Can you work these out from the model? Positions are in its coordinate system, mm. A direction names the side the tool comes from. Round coordinates to 2 decimals unless told otherwise and drop trailing zeros. Loops run counter-clockwise (first coordinate to the right, second up) from the corner with the lowest first, then second, coordinate; pieces in that order, holes last.
from build123d import *

# Parameters (mm, degrees)
ESQUISSE1_W                                    = 408.5
ESQUISSE1_H                                    = 181
BOSS_EXTRU_1_DEPTH                             = 8
CHAMBRAGE_POUR_VIS_T_TE_RONDE_BOMB_2_COUNT     = 2
CHAMBRAGE_POUR_VIS_T_TE_RONDE_BOMB_2_PITCH     = 56
CHAMBRAGE_POUR_VIS_T_TE_RONDE_BOMB_3_COUNT     = 2
CHAMBRAGE_POUR_VIS_T_TE_RONDE_BOMB_3_PITCH     = 140
R_P_TITION_LIN_AIRE1_COUNT                     = 11
R_P_TITION_LIN_AIRE1_PITCH                     = 33
ESQUISSE4_W                                    = 22.5
ESQUISSE4_H                                    = 4.5
ENL_V_MAT_EXTRU_1_DEPTH                        = 181
ESQUISSE5_W                                    = 22.5
ESQUISSE5_H                                    = 18.725
BOSS_EXTRU_2_DEPTH                             = 3.5
ESQUISSE7_W                                    = 274.5
ESQUISSE7_H                                    = 22.375
BOSS_EXTRU_3_DEPTH                             = 5
FRAISAGE_POUR_VIS_T_TE_FRAIS_E_M31_D           = 3.4
FRAISAGE_POUR_VIS_T_TE_FRAIS_E_M31_CSINK_D     = 6.3
FRAISAGE_POUR_VIS_T_TE_FRAIS_E_M31_CSINK_ANGLE = 90
ESQUISSE10_W                                   = 204.25
ESQUISSE10_H                                   = 203.375
ENL_V_MAT_EXTRU_2_DEPTH                        = 10


with BuildPart() as part:
    # Esquisse1 → Boss.-Extru.1 (new body)
    with BuildSketch(Plane.XY):
        Rectangle(ESQUISSE1_W, ESQUISSE1_H)
    extrude(amount=BOSS_EXTRU_1_DEPTH)

    # Esquisse3 → Chambrage pour vis à tête ronde bombée M31 (revolve, cut)
    with BuildSketch(Plane(origin=(-156.75, 63, 8), x_dir=(0, -1, 0), z_dir=(1, 0, 0))):
        Polygon((0, 0), (0, 8), (1.6, 8), (1.6, 2.4), (3.5, 2.4), (3.5, 0.025), (3.525, 0), align=None)
    chambrage_pour_vis_t_te_ronde_bomb_e_m = revolve(axis=Axis((-156.75, 63, 14.35), (0, 0, -1)), mode=Mode.SUBTRACT)

    # Chambrage pour vis _ t_te ronde bomb 2: Chambrage pour vis à tête ronde bombée M31 ×2
    with Locations(*[(0, -i * CHAMBRAGE_POUR_VIS_T_TE_RONDE_BOMB_2_PITCH, 0) for i in range(1, CHAMBRAGE_POUR_VIS_T_TE_RONDE_BOMB_2_COUNT)]):
        add(chambrage_pour_vis_t_te_ronde_bomb_e_m, mode=Mode.SUBTRACT)

    # Chambrage pour vis _ t_te ronde bomb 3: Chambrage pour vis à tête ronde bombée M31 ×2
    with Locations(*[(0, -i * CHAMBRAGE_POUR_VIS_T_TE_RONDE_BOMB_3_PITCH, 0) for i in range(1, CHAMBRAGE_POUR_VIS_T_TE_RONDE_BOMB_3_COUNT)]):
        add(chambrage_pour_vis_t_te_ronde_bomb_e_m, mode=Mode.SUBTRACT)

    # Répétition linéaire1: Chambrage pour vis à tête ronde bombée M31 ×11
    with Locations(*[(i * R_P_TITION_LIN_AIRE1_PITCH, 0, 0) for i in range(1, R_P_TITION_LIN_AIRE1_COUNT)]):
        add(chambrage_pour_vis_t_te_ronde_bomb_e_m, mode=Mode.SUBTRACT)

    # Répétition linéaire1 copy 1 sketch → Répétition linéaire1 copy 1 (revolve, cut)
    with BuildSketch(Plane(origin=(-123.75, 7, 8), x_dir=(0, -1, 0), z_dir=(1, 0, 0))):
        Polygon((0, 0), (0, 8), (1.6, 8), (1.6, 2.4), (3.5, 2.4), (3.5, 0.025), (3.525, 0), align=None)
    revolve(axis=Axis((-123.75, 7, 14.35), (0, 0, -1)), mode=Mode.SUBTRACT)

    # Répétition linéaire1 copy 2 sketch → Répétition linéaire1 copy 2 (revolve, cut)
    with BuildSketch(Plane(origin=(-90.75, 7, 8), x_dir=(0, -1, 0), z_dir=(1, 0, 0))):
        Polygon((0, 0), (0, 8), (1.6, 8), (1.6, 2.4), (3.5, 2.4), (3.5, 0.025), (3.525, 0), align=None)
    revolve(axis=Axis((-90.75, 7, 14.35), (0, 0, -1)), mode=Mode.SUBTRACT)

    # Répétition linéaire1 copy 3 sketch → Répétition linéaire1 copy 3 (revolve, cut)
    with BuildSketch(Plane(origin=(-57.75, 7, 8), x_dir=(0, -1, 0), z_dir=(1, 0, 0))):
        Polygon((0, 0), (0, 8), (1.6, 8), (1.6, 2.4), (3.5, 2.4), (3.5, 0.025), (3.525, 0), align=None)
    revolve(axis=Axis((-57.75, 7, 14.35), (0, 0, -1)), mode=Mode.SUBTRACT)

    # Répétition linéaire1 copy 4 sketch → Répétition linéaire1 copy 4 (revolve, cut)
    with BuildSketch(Plane(origin=(-24.75, 7, 8), x_dir=(0, -1, 0), z_dir=(1, 0, 0))):
        Polygon((0, 0), (0, 8), (1.6, 8), (1.6, 2.4), (3.5, 2.4), (3.5, 0.025), (3.525, 0), align=None)
    revolve(axis=Axis((-24.75, 7, 14.35), (0, 0, -1)), mode=Mode.SUBTRACT)

    # Répétition linéaire1 copy 5 sketch → Répétition linéaire1 copy 5 (revolve, cut)
    with BuildSketch(Plane(origin=(8.25, 7, 8), x_dir=(0, -1, 0), z_dir=(1, 0, 0))):
        Polygon((0, 0), (0, 8), (1.6, 8), (1.6, 2.4), (3.5, 2.4), (3.5, 0.025), (3.525, 0), align=None)
    revolve(axis=Axis((8.25, 7, 14.35), (0, 0, -1)), mode=Mode.SUBTRACT)

    # Répétition linéaire1 copy 6 sketch → Répétition linéaire1 copy 6 (revolve, cut)
    with BuildSketch(Plane(origin=(41.25, 7, 8), x_dir=(0, -1, 0), z_dir=(1, 0, 0))):
        Polygon((0, 0), (0, 8), (1.6, 8), (1.6, 2.4), (3.5, 2.4), (3.5, 0.025), (3.525, 0), align=None)
    revolve(axis=Axis((41.25, 7, 14.35), (0, 0, -1)), mode=Mode.SUBTRACT)

    # Répétition linéaire1 copy 7 sketch → Répétition linéaire1 copy 7 (revolve, cut)
    with BuildSketch(Plane(origin=(74.25, 7, 8), x_dir=(0, -1, 0), z_dir=(1, 0, 0))):
        Polygon((0, 0), (0, 8), (1.6, 8), (1.6, 2.4), (3.5, 2.4), (3.5, 0.025), (3.525, 0), align=None)
    revolve(axis=Axis((74.25, 7, 14.35), (0, 0, -1)), mode=Mode.SUBTRACT)

    # Répétition linéaire1 copy 8 sketch → Répétition linéaire1 copy 8 (revolve, cut)
    with BuildSketch(Plane(origin=(107.25, 7, 8), x_dir=(0, -1, 0), z_dir=(1, 0, 0))):
        Polygon((0, 0), (0, 8), (1.6, 8), (1.6, 2.4), (3.5, 2.4), (3.5, 0.025), (3.525, 0), align=None)
    revolve(axis=Axis((107.25, 7, 14.35), (0, 0, -1)), mode=Mode.SUBTRACT)

    # Répétition linéaire1 copy 9 sketch → Répétition linéaire1 copy 9 (revolve, cut)
    with BuildSketch(Plane(origin=(140.25, 7, 8), x_dir=(0, -1, 0), z_dir=(1, 0, 0))):
        Polygon((0, 0), (0, 8), (1.6, 8), (1.6, 2.4), (3.5, 2.4), (3.5, 0.025), (3.525, 0), align=None)
    revolve(axis=Axis((140.25, 7, 14.35), (0, 0, -1)), mode=Mode.SUBTRACT)

    # Répétition linéaire1 copy 10 sketch → Répétition linéaire1 copy 10 (revolve, cut)
    with BuildSketch(Plane(origin=(173.25, 7, 8), x_dir=(0, -1, 0), z_dir=(1, 0, 0))):
        Polygon((0, 0), (0, 8), (1.6, 8), (1.6, 2.4), (3.5, 2.4), (3.5, 0.025), (3.525, 0), align=None)
    revolve(axis=Axis((173.25, 7, 14.35), (0, 0, -1)), mode=Mode.SUBTRACT)

    # Répétition linéaire1 copy 11 sketch → Répétition linéaire1 copy 11 (revolve, cut)
    with BuildSketch(Plane(origin=(-123.75, -77, 8), x_dir=(0, -1, 0), z_dir=(1, 0, 0))):
        Polygon((0, 0), (0, 8), (1.6, 8), (1.6, 2.4), (3.5, 2.4), (3.5, 0.025), (3.525, 0), align=None)
    revolve(axis=Axis((-123.75, -77, 14.35), (0, 0, -1)), mode=Mode.SUBTRACT)

    # Répétition linéaire1 copy 12 sketch → Répétition linéaire1 copy 12 (revolve, cut)
    with BuildSketch(Plane(origin=(-90.75, -77, 8), x_dir=(0, -1, 0), z_dir=(1, 0, 0))):
        Polygon((0, 0), (0, 8), (1.6, 8), (1.6, 2.4), (3.5, 2.4), (3.5, 0.025), (3.525, 0), align=None)
    revolve(axis=Axis((-90.75, -77, 14.35), (0, 0, -1)), mode=Mode.SUBTRACT)

    # Répétition linéaire1 copy 13 sketch → Répétition linéaire1 copy 13 (revolve, cut)
    with BuildSketch(Plane(origin=(-57.75, -77, 8), x_dir=(0, -1, 0), z_dir=(1, 0, 0))):
        Polygon((0, 0), (0, 8), (1.6, 8), (1.6, 2.4), (3.5, 2.4), (3.5, 0.025), (3.525, 0), align=None)
    revolve(axis=Axis((-57.75, -77, 14.35), (0, 0, -1)), mode=Mode.SUBTRACT)

    # Répétition linéaire1 copy 14 sketch → Répétition linéaire1 copy 14 (revolve, cut)
    with BuildSketch(Plane(origin=(-24.75, -77, 8), x_dir=(0, -1, 0), z_dir=(1, 0, 0))):
        Polygon((0, 0), (0, 8), (1.6, 8), (1.6, 2.4), (3.5, 2.4), (3.5, 0.025), (3.525, 0), align=None)
    revolve(axis=Axis((-24.75, -77, 14.35), (0, 0, -1)), mode=Mode.SUBTRACT)

    # Répétition linéaire1 copy 15 sketch → Répétition linéaire1 copy 15 (revolve, cut)
    with BuildSketch(Plane(origin=(8.25, -77, 8), x_dir=(0, -1, 0), z_dir=(1, 0, 0))):
        Polygon((0, 0), (0, 8), (1.6, 8), (1.6, 2.4), (3.5, 2.4), (3.5, 0.025), (3.525, 0), align=None)
    revolve(axis=Axis((8.25, -77, 14.35), (0, 0, -1)), mode=Mode.SUBTRACT)

    # Répétition linéaire1 copy 16 sketch → Répétition linéaire1 copy 16 (revolve, cut)
    with BuildSketch(Plane(origin=(41.25, -77, 8), x_dir=(0, -1, 0), z_dir=(1, 0, 0))):
        Polygon((0, 0), (0, 8), (1.6, 8), (1.6, 2.4), (3.5, 2.4), (3.5, 0.025), (3.525, 0), align=None)
    revolve(axis=Axis((41.25, -77, 14.35), (0, 0, -1)), mode=Mode.SUBTRACT)

    # Répétition linéaire1 copy 17 sketch → Répétition linéaire1 copy 17 (revolve, cut)
    with BuildSketch(Plane(origin=(74.25, -77, 8), x_dir=(0, -1, 0), z_dir=(1, 0, 0))):
        Polygon((0, 0), (0, 8), (1.6, 8), (1.6, 2.4), (3.5, 2.4), (3.5, 0.025), (3.525, 0), align=None)
    revolve(axis=Axis((74.25, -77, 14.35), (0, 0, -1)), mode=Mode.SUBTRACT)

    # Répétition linéaire1 copy 18 sketch → Répétition linéaire1 copy 18 (revolve, cut)
    with BuildSketch(Plane(origin=(107.25, -77, 8), x_dir=(0, -1, 0), z_dir=(1, 0, 0))):
        Polygon((0, 0), (0, 8), (1.6, 8), (1.6, 2.4), (3.5, 2.4), (3.5, 0.025), (3.525, 0), align=None)
    revolve(axis=Axis((107.25, -77, 14.35), (0, 0, -1)), mode=Mode.SUBTRACT)

    # Répétition linéaire1 copy 19 sketch → Répétition linéaire1 copy 19 (revolve, cut)
    with BuildSketch(Plane(origin=(140.25, -77, 8), x_dir=(0, -1, 0), z_dir=(1, 0, 0))):
        Polygon((0, 0), (0, 8), (1.6, 8), (1.6, 2.4), (3.5, 2.4), (3.5, 0.025), (3.525, 0), align=None)
    revolve(axis=Axis((140.25, -77, 14.35), (0, 0, -1)), mode=Mode.SUBTRACT)

    # Répétition linéaire1 copy 20 sketch → Répétition linéaire1 copy 20 (revolve, cut)
    with BuildSketch(Plane(origin=(173.25, -77, 8), x_dir=(0, -1, 0), z_dir=(1, 0, 0))):
        Polygon((0, 0), (0, 8), (1.6, 8), (1.6, 2.4), (3.5, 2.4), (3.5, 0.025), (3.525, 0), align=None)
    revolve(axis=Axis((173.25, -77, 14.35), (0, 0, -1)), mode=Mode.SUBTRACT)

    # Esquisse4 → Enlèv. mat.-Extru.1 (cut)
    with BuildSketch(Plane(origin=(0, 90.5, 0), x_dir=(1, 0, 0), z_dir=(0, 1, 0))):
        with Locations((-193, -2.25)):
            Rectangle(ESQUISSE4_W, ESQUISSE4_H)
        with Locations((193, -2.25)):
            Rectangle(ESQUISSE4_W, ESQUISSE4_H)
    extrude(amount=-ENL_V_MAT_EXTRU_1_DEPTH, mode=Mode.SUBTRACT)

    # Esquisse5 → Boss.-Extru.2 (add)
    with BuildSketch(Plane.XY.offset(8)):
        with Locations((-193, 99.8625)):
            Rectangle(ESQUISSE5_W, ESQUISSE5_H)
    boss_extru_2 = extrude(amount=-BOSS_EXTRU_2_DEPTH)

    # Symétrie1: Boss.-Extru.2 across plane
    add(boss_extru_2.mirror(Plane(origin=(0, 0, 0), x_dir=(0, 0, 1), z_dir=(1, 0, 0))))

    # Esquisse7 → Boss.-Extru.3 (add)
    with BuildSketch(Plane.XY.offset(8)):
        with Locations((0, 101.6875)):
            Rectangle(ESQUISSE7_W, ESQUISSE7_H)
    extrude(amount=-BOSS_EXTRU_3_DEPTH)

    # Fraisage pour vis à tête fraisée M31 (through all)
    with Locations(Plane.XY.offset(8)):
        with Locations((-131.25, 98), (131.25, 98)):
            CounterSinkHole(FRAISAGE_POUR_VIS_T_TE_FRAIS_E_M31_D / 2, FRAISAGE_POUR_VIS_T_TE_FRAIS_E_M31_CSINK_D / 2, counter_sink_angle=FRAISAGE_POUR_VIS_T_TE_FRAIS_E_M31_CSINK_ANGLE)

    # Esquisse10 → Enlèv. mat.-Extru.2 (cut)
    with BuildSketch(Plane(origin=(0, 0, 0), x_dir=(-1, 0, 0), z_dir=(0, 0, -1))):
        with Locations((102.125, 11.1875)):
            Rectangle(ESQUISSE10_W, ESQUISSE10_H)
    extrude(amount=-ENL_V_MAT_EXTRU_2_DEPTH, mode=Mode.SUBTRACT)


solid = part.part
(1) Will these pins go through, and if not, where does the flat tip stop? P1, Ø6.5, axis at x = 82, y = 103, coming from the -Z side; P2, Ø4, axis at x = 166, z = 3, coming from the +Y side; P3, Ø5, axis at x = 74.25, y = 7, coming from the +Z side.
Worked answers:
P1: stops at z = 3
P2: stops at y = 90.5
P3: stops at z = 5.6
(2) For faces 1 (the flat face through (137.25, 102, 6)), 2 (the flat face through (9, -75, 5.6)), which set-ups out of +Z, -Z, +X, -X, +Y, -Y let a thin tool reach every point of the face, with its end or its side?
Worked answers:
face 1: +Z, -Z, +Y
face 2: +Z
(3) If we section it at C-C, the plane x = 157.5: List the corners of the cut face in (y, z) for me.
Worked answers:
outline: (-90.5, 0) - (90.5, 0) - (90.5, 8) - (-90.5, 8) - close
(4) If we mould it in two halves opening along X, with no side actions, what happens to faces 3 (the flat face through (0, 10, 4)), 4 (the flat face through (141, 65, 5.6)), 5 (the flat face through (90, 1, 0))? For each: released by +X, released by -X, zero draft, split by the parting line, or undercut.
Worked answers:
face 3: released by -X
face 4: undercut
face 5: zero draft
(5) If we section it at A-A, the plane x = 25: List the corners of the cut face in (y, z) for me (3 decimals), then the cut area to 3 significant figures.
Worked answers:
outline: (-90.5, 0) - (90.5, 0) - (90.5, 3) - (112.875, 3) - (112.875, 8) - (-90.5, 8) - close
area: 1,560 mm2
(6) If we section it at B-B, the plane y = -6: List the corners of the cut face in (x, z) for me, then the cut area to 3 significant figures.
Worked answers:
outline: (0, 0) - (181.75, 0) - (181.75, 4.5) - (204.25, 4.5) - (204.25, 8) - (0, 8) - close
area: 1,530 mm2
(7) If I drill on line 1 (Y direction, x = 173.25, z = 7.4); line 2 (Y direction, x = 107.25, z = 4.35) (3 decimals); line 3 (Y direction, x = 163, z = 4), over which ranges is the centre line in solid material (lowest first)?
Worked answers:
line 1: y = -90.5 to -80.5, -73.5 to 3.5, 10.5 to 59.5, 66.5 to 90.5
line 2: y = -90.5 to -78.6, -75.4 to 5.4, 8.6 to 61.4, 64.6 to 112.875
line 3: y = -90.5 to 90.5
